from build123d import *

# Parameters (mm, degrees)
BOSS_EXTRUDE1_DEPTH = 44.4
SKETCH4_R           = 2.6
CUT_EXTRUDE1_DEPTH  = 59.211840581
SKETCH6_R           = 2.6
CUT_EXTRUDE2_DEPTH  = 65.569616831
CHAMFER1_SIZE       = 2
SKETCH7_R           = 2.6
CUT_EXTRUDE3_DEPTH  = 59.43220581
SKETCH9_R           = 2.6
CUT_EXTRUDE4_DEPTH  = 60.570802035


with BuildPart() as part:
    # Sketch1 → Boss-Extrude1 (new body)
    with BuildSketch(Plane.XY):
        Polygon((-23.440752002, -3.891774983), (-8.35, 4.820874748), (-8.35, 22.246174209), (8.35, 22.246174209), (8.35, 4.820874748), (23.440752002, -3.891774983), (15.090752002, -18.354399226), (0, -9.641749495), (-15.090752002, -18.354399226), align=None)
        Polygon((20.708701195, -4.623825791), (6.35, 3.666174209), (6.35, 20.246174209), (-6.35, 20.246174209), (-6.35, 3.666174209), (-20.708701195, -4.623825791), (-14.358701195, -15.622348419), (0, -7.332348419), (14.358701195, -15.622348419), align=None, mode=Mode.SUBTRACT)
    extrude(amount=BOSS_EXTRUDE1_DEPTH)

    # Sketch4 → Cut-Extrude1 (cut, through all)
    with BuildSketch(Plane(origin=(-4.175, 7.231312122, 0), x_dir=(0.8660254037844606, 0.4999999999999621, 0), z_dir=(-0.4999999999999621, 0.8660254037844606, 0))):
        with Locations(Location((-11.644441584, -10, 0), (0, 0, 180))):
            Circle(SKETCH4_R)
        with Locations(Location((-11.644441584, -34.4, 0), (0, 0, 180))):
            Circle(SKETCH4_R)
    extrude(amount=-CUT_EXTRUDE1_DEPTH, mode=Mode.SUBTRACT)

    # Sketch6 → Cut-Extrude2 (cut, through all)
    with BuildSketch(Plane(origin=(0, 22.246174209, 0), x_dir=(1, 0, 0), z_dir=(0, 1, 0))):
        with Locations(Location((0, -12.2, 0), (0, 0, 270))):
            Circle(SKETCH6_R)
        with Locations(Location((0, -32.2, 0), (0, 0, 270))):
            Circle(SKETCH6_R)
    extrude(amount=-CUT_EXTRUDE2_DEPTH, mode=Mode.SUBTRACT)

    # Chamfer1
    # the kernel refuses this chamfer: 2 mm, written as the material it adds along each edge
    with BuildSketch(Plane(origin=(-8.35, 4.820874748, 0), x_dir=(-0.8562002652919762, -0.516644080304758, 0), z_dir=(0, 0, 1)), Plane(origin=(8.35, 4.820874748, 0), x_dir=(-0.019326765612699432, 0.9998132206222079, 0), z_dir=(0, 0, 1))) as chamfer1_piece_1:
        Polygon((CHAMFER1_SIZE * 0.999813220622, -CHAMFER1_SIZE * 0.0193267656127), (-CHAMFER1_SIZE * 0.516644080305, -CHAMFER1_SIZE * 0.856200265292), (0, 0), align=None)
    extrude(amount=44.4)
    with BuildSketch(Plane(origin=(0, -9.641749495, 0), x_dir=(-0.8755270309047186, -0.48316914031751634, 0), z_dir=(0, 0, 1))) as chamfer1_piece_2_section:
        Polygon((CHAMFER1_SIZE * 0.999813220622, CHAMFER1_SIZE * 0.0193267656127), (-CHAMFER1_SIZE * 0.516644080305, CHAMFER1_SIZE * 0.856200265292), (0, 0), align=None)
    chamfer1_piece_2 = extrude(amount=14.774171509, mode=Mode.PRIVATE)
    chamfer1_piece_2 = chamfer1_piece_2 - Plane(origin=(0, -10.299671393, 12.2), x_dir=(0, 0, 1), z_dir=(0, 1, 0)) * Cylinder(2.6, 38, mode=Mode.PRIVATE)
    add(chamfer1_piece_2)
    with BuildSketch(Plane(origin=(0, -9.641749495, 9.625828491), x_dir=(-0.8755270309047187, -0.48316914031751634, 0), z_dir=(0, 0, 1))) as chamfer1_piece_3_section:
        Polygon((CHAMFER1_SIZE * 0.999813220622, CHAMFER1_SIZE * 0.0193267656127), (-CHAMFER1_SIZE * 0.516644080305, CHAMFER1_SIZE * 0.856200265292), (0, 0), align=None)
    chamfer1_piece_3 = extrude(amount=25.148343019, mode=Mode.PRIVATE)
    chamfer1_piece_3 = chamfer1_piece_3 - Plane(origin=(0, -10.461752063, 32.2), x_dir=(0, 0, 1), z_dir=(0, 1, 0)) * Cylinder(2.6, 59, mode=Mode.PRIVATE)
    chamfer1_piece_3 = chamfer1_piece_3 - Plane(origin=(0, -10.461752063, 12.2), x_dir=(0, 0, 1), z_dir=(0, 1, 0)) * Cylinder(2.6, 59, mode=Mode.PRIVATE)
    add(chamfer1_piece_3)
    with BuildSketch(Plane(origin=(0, -9.641749495, 29.625828491), x_dir=(-0.8755270309047187, -0.48316914031751634, 0), z_dir=(0, 0, 1))) as chamfer1_piece_4_section:
        Polygon((CHAMFER1_SIZE * 0.999813220622, CHAMFER1_SIZE * 0.0193267656127), (-CHAMFER1_SIZE * 0.516644080305, CHAMFER1_SIZE * 0.856200265292), (0, 0), align=None)
    chamfer1_piece_4 = extrude(amount=14.774171509, mode=Mode.PRIVATE)
    chamfer1_piece_4 = chamfer1_piece_4 - Plane(origin=(0, -10.461752063, 32.2), x_dir=(0, 0, 1), z_dir=(0, 1, 0)) * Cylinder(2.6, 38, mode=Mode.PRIVATE)
    add(chamfer1_piece_4)
    # the kernel refuses this chamfer: 2 mm, written as the material it takes off along each edge
    with BuildSketch(Plane(origin=(-8.35, 22.246174209, -5.143365976), x_dir=(0.9996219169112968, 0.027495876610585623, 0), z_dir=(0, 0, 1)), Plane(origin=(8.35, 22.246174209, -5.143365976), x_dir=(0.02749587661058651, -0.9996219169112968, 0), z_dir=(0, 0, 1)), Plane(origin=(23.440752002, -3.891774983, -5.143365976), x_dir=(-0.4759988308116281, -0.8794459125301357, 0), z_dir=(0, 0, 1)), Plane(origin=(15.090752002, -18.354399226, -5.143365976), x_dir=(-0.8794459125301354, 0.4759988308116286, 0), z_dir=(0, 0, 1)), Plane(origin=(-23.440752002, -3.891774983, -5.143365976), x_dir=(0.851950035919547, 0.5236230860998039, 0), z_dir=(0, 0, 1))) as chamfer1_2_piece_1:
        Polygon((CHAMFER1_SIZE * 0.999621916911, -CHAMFER1_SIZE * 0.0274958766106), (-CHAMFER1_SIZE * 0.0274958766106, -CHAMFER1_SIZE * 0.999621916911), (0, 0), align=None)
    extrude(amount=54.686731952, mode=Mode.SUBTRACT)
    with BuildSketch(Plane(origin=(-15.090752002, -18.354399226, -5.143365976), x_dir=(0.8794459125301743, 0.4759988308115566, 0), z_dir=(0, 0, 1))) as chamfer1_2_piece_2:
        Polygon((CHAMFER1_SIZE * 0.999621916911, CHAMFER1_SIZE * 0.0274958766106), (-CHAMFER1_SIZE * 0.0274958766105, CHAMFER1_SIZE * 0.999621916911), (0, 0), align=None)
    extrude(amount=54.686731952, mode=Mode.SUBTRACT)

    # Sketch7 → Cut-Extrude3 (cut, through all)
    with BuildSketch(Plane(origin=(8.35, 0, 0), x_dir=(0, 0, -1), z_dir=(1, 0, 0))):
        with Locations((-10, 11.644441584)):
            Circle(SKETCH7_R)
        with Locations((-34.4, 11.644441584)):
            Circle(SKETCH7_R)
    extrude(amount=-CUT_EXTRUDE3_DEPTH, mode=Mode.SUBTRACT)

    # Sketch9 → Cut-Extrude4 (cut, through all)
    with BuildSketch(Plane(origin=(-4.175, -7.231312122, 0), x_dir=(0.8660254037844506, -0.49999999999997924, 0), z_dir=(-0.4999999999999793, -0.8660254037844507, 0))):
        with Locations((11.644441584, 34.4)):
            Circle(SKETCH9_R)
        with Locations((11.644441584, 10)):
            Circle(SKETCH9_R)
    extrude(amount=-CUT_EXTRUDE4_DEPTH, mode=Mode.SUBTRACT)


solid = part.part
The listing builds one solid part. Answer for the finished solid, in the listing's coordinates (mm). A direction names the side the tool comes from. Round coordinates to 2 decimals unless told otherwise and drop trailing zeros. Order: outer loops, then holes, each group sorted by start corner. A loop starts at its lowest first (then second) coordinate and runs counter-clockwise, first axis right, second up. Notation, with made-up numbers: (-30.5, 75.25) -> (13.5, 75.25) arc R18 ccw to (13.5, 102.25) -> close; hole circle Ø2 at (71, 30.5). An arc over 180 degrees is marked (long way). Put each result on its own line as item: value.
Q1. Section A-A, the plane z = 24 is taken. Write down the section's boundary in (x, y).
Results list:
outline: (-22.44, -5.62) -> (-16.09, -16.62) -> (-13.36, -17.35) -> (-1.73, -10.64) -> (1.73, -10.64) -> (13.36, -17.35) -> (16.09, -16.62) -> (22.44, -5.62) -> (21.71, -2.89) -> (10.08, 3.82) -> (8.35, 6.82) -> (8.35, 20.25) -> (6.35, 22.25) -> (-6.35, 22.25) -> (-8.35, 20.25) -> (-8.35, 6.82) -> (-10.08, 3.82) -> (-21.71, -2.89) -> close; hole (-20.71, -4.62) -> (-14.36, -15.62) -> (0, -7.33) -> (14.36, -15.62) -> (20.71, -4.62) -> (6.35, 3.67) -> (6.35, 20.25) -> (-6.35, 20.25) -> (-6.35, 3.67) -> close
Q2. Each of these flat-tipped pins is pushed along its axis until it touches: P1, Ø6, axis at x = 0, z = 12.2, coming from the -Y side; P2, Ø18, axis at y = 16, z = 29, coming from the +X side; P3, Ø4, axis at y = 3.5, z = 25, coming from the -X side. Where does it stop, or does it pass through?
Results list:
P1: y = -11.37
P2: x = 8.35
P3: x = -14.1
Q3. Determine the mould class of faces 1 (the cylindrical face through (-7.34, 9.34, 8.8)), 2 (the flat face through (19.31, -11.05, 21.89)), 3 (the flat face through (0, -8, 0)) for opening direction Z: pulls with the +Z half, pulls with the -Z half, needs draft (parallel to the pull), parting line crosses it, or undercut.
Results list:
face 1: undercut
face 2: needs draft
face 3: pulls with the -Z half
Q4. Section B-B, the plane x = -18 is taken. Write down the section's boundary in (y, z).
Results list:
outline: (-13.32, 0) -> (-9.32, 0) -> (-9.32, 44.4) -> (-13.32, 44.4) -> close; (-3.06, 0) -> (-0.75, 0) -> (-0.75, 44.4) -> (-3.06, 44.4) -> close
Q5. Section D-D, the plane x = 5.5 is taken. Count the separate pieces of the cut face and the enclosed holes in it, and give its area (3 significant figures).
Results list:
separate pieces: 4
enclosed holes: 0
area: 170 mm^2
Q6. Section C-C, the plane y = 13 is taken. Write down the section's boundary in (x, z), and give its area (3 significant figures).
Results list:
outline: (-8.35, 0) -> (-6.35, 0) -> (-6.35, 7.78) -> (-8.35, 7.78) -> close; (-8.35, 12.22) -> (-6.35, 12.22) -> (-6.35, 32.18) -> (-8.35, 32.18) -> close; (-8.35, 36.62) -> (-6.35, 36.62) -> (-6.35, 44.4) -> (-8.35, 44.4) -> close; (6.35, 0) -> (8.35, 0) -> (8.35, 7.78) -> (6.35, 7.78) -> close; (6.35, 12.22) -> (8.35, 12.22) -> (8.35, 32.18) -> (6.35, 32.18) -> close; (6.35, 36.62) -> (8.35, 36.62) -> (8.35, 44.4) -> (6.35, 44.4) -> close
area: 142 mm^2
Q7. Consider line 1 along X through (y, z) = (12, 19); line 2 along X through (y, z) = (-13.5, 23). Determine where each line is inside the solid, lowest interval first.
Results list:
line 1: -8.35 to -6.35, 6.35 to 8.35
line 2: -17.89 to -15.58, -10.68 to -6.68, 6.68 to 10.68, 15.58 to 17.89
Q8. Which of the six approach directions +Z, -Z, +X, -X, +Y, -Y give full straight-line access (tool end or side, diameter ignored) to faces 4 (the flat face through (-14.706, -16.993, 21.889)), 5 (the flat face through (-17.578, -10.046, 21.889)), 6 (the flat face through (0, -10.642, 22))?
Results list:
face 4: +Z, -Z, -X, -Y
face 5: +Z, -Z
face 6: +Z, -Z, -Y
